For this review, take the finished solid that the model builds, in its own axes (mm). Coordinates: 2 decimals unless noted, no trailing zeros. Write each loop counter-clockwise with the first axis right and the second up, starting at its lowest first coordinate (ties: lowest second). Pieces come first, ordered by that corner, then holes.
```python
from build123d import *

# Parameters (mm, degrees)
SKETCH1_R           = 1.42
SKETCH1_W           = 7
SKETCH1_H           = 4
BOSS_EXTRUDE2_DEPTH = 3


with BuildPart() as part:
    # Sketch1 → Boss-Extrude2 (new body)
    with BuildSketch(Plane.XY):
        Polygon((36.149381, 0), (36.149381, -3), (52.149381, -3), (52.149381, 0), (106.959381, 0), (106.959381, -3), (122.959381, -3), (122.959381, 0), (141.38, 0), (141.38, 27.105503225), (141.38, 85.806519795), (140.170833607, 85.806519795), (122.959381, 85.806519795), (106.959381, 85.806519795), (0, 12.520138185), (0, 0), align=None)
        with Locations((44.149381, -1.5)):
            Circle(SKETCH1_R, mode=Mode.SUBTRACT)
        with Locations((114.959381, -1.5)):
            Circle(SKETCH1_R, mode=Mode.SUBTRACT)
        Polygon((20.433228311, 12.520138185), (99.128706317, 67.278357703), (106.959381, 72.806519795), (106.959381, 12.520138185), (99.128706317, 12.520138185), align=None, mode=Mode.SUBTRACT)
        with Locations((127.88, 70.806519795)):
            Rectangle(SKETCH1_W, SKETCH1_H, mode=Mode.SUBTRACT)
        with Locations((127.88, 79.806519795)):
            Rectangle(SKETCH1_W, SKETCH1_H, mode=Mode.SUBTRACT)
        with Locations((127.88, 61.806519795)):
            Rectangle(SKETCH1_W, SKETCH1_H, mode=Mode.SUBTRACT)
        with Locations((127.88, 52.806519795)):
            Rectangle(SKETCH1_W, SKETCH1_H, mode=Mode.SUBTRACT)
        with Locations((127.88, 43.806519795)):
            Rectangle(SKETCH1_W, SKETCH1_H, mode=Mode.SUBTRACT)
        with Locations((127.88, 34.806519795)):
            Rectangle(SKETCH1_W, SKETCH1_H, mode=Mode.SUBTRACT)
        with Locations((127.88, 25.806519795)):
            Rectangle(SKETCH1_W, SKETCH1_H, mode=Mode.SUBTRACT)
        with Locations((127.88, 16.806519795)):
            Rectangle(SKETCH1_W, SKETCH1_H, mode=Mode.SUBTRACT)
    extrude(amount=BOSS_EXTRUDE2_DEPTH)


solid = part.part
```
Q1. Add section B-B (x = 38.5). State the section outline as (y, z) points, then the cut area to 3 significant figures.
Ans:
outline: (-3, 0) - (12.52, 0) - (12.52, 3) - (-3, 3) - close; (25.09, 0) - (38.9, 0) - (38.9, 3) - (25.09, 3) - close
area: 88.0 mm2
Q2. Add section A-A (y = -1.5). State the section outline as (x, z) points, then the cut area to 3 significant figures.
Ans:
outline: (36.15, 0) - (42.73, 0) - (42.73, 3) - (36.15, 3) - close; (45.57, 0) - (52.15, 0) - (52.15, 3) - (45.57, 3) - close; (106.96, 0) - (113.54, 0) - (113.54, 3) - (106.96, 3) - close; (116.38, 0) - (122.96, 0) - (122.96, 3) - (116.38, 3) - close
area: 79.0 mm2
Q3. Add section D-D (z = 1.05). Give the number of separate pieces and of enclosed holes in the cut face, then the cut area to 3 significant figures.
Ans:
separate pieces: 1
enclosed holes: 11
area: 5,470 mm2
Q4. Add section C-C (y = 31). State the section outline as (x, z) points, then the cut area to 3 significant figures.
Ans:
outline: (26.97, 0) - (46.99, 0) - (46.99, 3) - (26.97, 3) - close; (106.96, 0) - (141.38, 0) - (141.38, 3) - (106.96, 3) - close
area: 163 mm2
Q5. For probe 1 along X at (y, z) = (52.5, 1.5); probe 2 along Y at (x, z) = (36, 0.8); probe 3 along Y at (x, z) = (99, 0.95), list the stretches that pass through material, from the lowest coordinate up.
Ans:
probe 1: x = 58.35 to 77.89, 106.96 to 124.38, 131.38 to 141.38
probe 2: y = 0 to 12.52, 23.35 to 37.19
probe 3: y = 0 to 12.52, 67.19 to 80.35
Q6. Clearance check with flat-ended pins moving along their axes: pin 1 Ø0.9 at (y, z) = (63, 1.5) entering from -X; pin 2 Ø0.9 at (y, z) = (-2, 1.5) entering from -X; pin 3 Ø0.9 at (x, z) = (126.5, 1) entering from -Y. State where each tip first meets the part, or that it passes through.
Ans:
pin 1: stops at x = 73.02
pin 2: stops at x = 36.15
pin 3: stops at y = 0
Q7. Draft analysis for pull direction Y (two halves, no side actions). For faces 1 (the flat face through (124, 85.807, 1)), 2 (the flat face through (106.959, -1, 1)), 3 (the flat face through (128, 45.807, 1)), state which applies: +Y half, -Y half, draft (parallel to the pull), parting line (faces both ways), or undercut.
Ans:
face 1: +Y half
face 2: draft
face 3: undercut
